```python
from build123d import *

# Parameters (mm, degrees)
CROQUIS1_W                       = 160
CROQUIS1_H                       = 140
CROQUIS1_R                       = 51.15
SALIENTE_EXTRUIR1_DEPTH          = 0.9
CROQUIS4_W                       = 20
CROQUIS4_H                       = 140
SALIENTE_EXTRUIR3_DEPTH          = 1
TALADRO_DE_MARGEN_PARA_M81_D     = 9
TALADRO_DE_MARGEN_PARA_M81_DEPTH = 10
TALADRO_DE_MARGEN_PARA_M81_TIP   = 2.703872786
SALIENTE_EXTRUIR4_DEPTH          = 21


with BuildPart() as part:
    # Croquis1 → Saliente-Extruir1 (new body)
    with BuildSketch(Plane(origin=(0, 0, 0), x_dir=(1, 0, 0), z_dir=(0, 1, 0))):
        Rectangle(CROQUIS1_W, CROQUIS1_H)
        with Locations(Location((0, 0, 0), (0, 0, 270))):
            Circle(CROQUIS1_R, mode=Mode.SUBTRACT)
    extrude(amount=SALIENTE_EXTRUIR1_DEPTH)

    # Croquis4 → Saliente-Extruir3 (add)
    with BuildSketch(Plane.XZ):
        with Locations((70, 0)):
            Rectangle(CROQUIS4_W, CROQUIS4_H)
        with Locations((-70, 0)):
            Rectangle(CROQUIS4_W, CROQUIS4_H)
    extrude(amount=SALIENTE_EXTRUIR3_DEPTH)

    # Taladro de margen para M81
    with Locations(Plane(origin=(-70, 0.9, -50), x_dir=(0, 0, 1), z_dir=(0, 1, 0))):
        with Locations((0, 0), (50, 0), (100, 0), (100, 140), (50, 140), (0, 140)):
            Hole(TALADRO_DE_MARGEN_PARA_M81_D / 2, depth=TALADRO_DE_MARGEN_PARA_M81_DEPTH)
            with Locations((0, 0, -(TALADRO_DE_MARGEN_PARA_M81_DEPTH + TALADRO_DE_MARGEN_PARA_M81_TIP / 2))):  # 118° drill point
                Cone(0, TALADRO_DE_MARGEN_PARA_M81_D / 2, TALADRO_DE_MARGEN_PARA_M81_TIP, mode=Mode.SUBTRACT)

    # Croquis5 → Saliente-Extruir4 (add)
    with BuildSketch(Plane.XZ):
        with BuildLine():
            ThreePointArc((57.15, 0), (0, 57.15), (-57.15, 0))
            Line((-57.15, 0), (-58.15, 0))
            ThreePointArc((-58.15, 0), (0, 58.15), (58.15, 0))
            Line((58.15, 0), (57.15, 0))
        make_face()
        with BuildLine():
            ThreePointArc((-58.141400912, -1), (0, -58.15), (58.141400912, -1))
            Line((58.141400912, -1), (57.141250424, -1))
            ThreePointArc((57.141250424, -1), (0, -57.15), (-57.141250424, -1))
            Line((-57.141250424, -1), (-58.141400912, -1))
        make_face()
    extrude(amount=-SALIENTE_EXTRUIR4_DEPTH)


solid = part.part
```
The model under review builds one solid part; all positions refer to its coordinate system, in mm. A direction names the side the tool comes from. Give positions to 0.01 mm unless a question says otherwise; leave off trailing zeros. Write each loop counter-clockwise with the first axis right and the second up, starting at its lowest first coordinate (ties: lowest second). Pieces come first, ordered by that corner, then holes. Notation, with made-up numbers: (20, -20.5) -> (37, -20.5) arc R18 ccw to (37, -6.5) -> close; hole circle Ø1 at (9.5, -36). An arc over 180 degrees is marked (long way). Put each result on its own line as item: value.
(1) Tool access review of faces 1 (the flat face through (41, 0, 32)), 2 (the cylindrical face through (1.257, 10.809, 57.136)), 3 (the cylindrical face through (-1.279, 10.809, 58.136)): name each direction out of +Z, -Z, +X, -X, +Y, -Y from which nothing blocks a thin tool from reaching the whole face with its end or side.
Results are:
face 1: +Z, -Z, -Y
face 2: +Y
face 3: +Z, +Y
(2) We need section B-B, the plane y = 4.75. Give the boundary of the cut face in (x, z).
Results are:
outline: (-58.15, 0) -> (-57.15, 0) arc R57.15 cw to (57.15, 0) -> (58.15, 0) arc R58.15 ccw to start; (-58.14, -1) arc R58.15 ccw to (58.14, -1) -> (57.14, -1) arc R57.15 cw to (-57.14, -1) -> close
(3) We need section C-C, the plane z = 2. Give the boundary of the cut face in (x, y) (3 decimals), and give its area (3 significant figures).
Results are:
outline: (-80, -1) -> (-74.031, -1) -> (-74.031, 0.9) -> (-80, 0.9) -> close; (-65.969, -1) -> (-60, -1) -> (-60, 0) -> (-51.111, 0) -> (-51.111, 0.9) -> (-57.115, 0.9) -> (-57.115, 21) -> (-58.116, 21) -> (-58.116, 0.9) -> (-65.969, 0.9) -> close; (51.111, 0) -> (60, 0) -> (60, -1) -> (65.969, -1) -> (65.969, 0.9) -> (58.116, 0.9) -> (58.116, 21) -> (57.115, 21) -> (57.115, 0.9) -> (51.111, 0.9) -> close; (74.031, -1) -> (80, -1) -> (80, 0.9) -> (74.031, 0.9) -> close
area: 102 mm²
(4) For pin 1 Ø4 at (y, z) = (13.5, 8.5) entering from -X; pin 2 Ø4 at (x, y) = (46.5, 11) entering from +Z; pin 3 Ø2 at (y, z) = (15.5, -51.5) entering from +X; pin 4 Ø7 at (x, z) = (70, 0) entering from +Y, all flat-tipped, find the tip position at first contact; note any pin that passes through.
Results are:
pin 1: x = -57.79
pin 2: z = 37.43
pin 3: x = 28.83
pin 4: through
(5) We need section A-A, the plane x = -70. Give the boundary of the cut face in (y, z).
Results are:
outline: (-1, -70) -> (0.9, -70) -> (0.9, -54.5) -> (-1, -54.5) -> close; (-1, -45.5) -> (0.9, -45.5) -> (0.9, -4.5) -> (-1, -4.5) -> close; (-1, 4.5) -> (0.9, 4.5) -> (0.9, 45.5) -> (-1, 45.5) -> close; (-1, 54.5) -> (0.9, 54.5) -> (0.9, 70) -> (-1, 70) -> close
(6) To check wall thickness, follow probe 1 along X at (y, z) = (-0.1, 0); probe 2 along Y at (x, z) = (49, -44.5); probe 3 along Z at (x, y) = (24, 17). State the ranges of each line that lie inside material, in increasing order. Write a range as from..to.
Results are:
probe 1: -80..-74.5, -65.5..-60, 60..65.5, 74.5..80
probe 2: 0..0.9
probe 3: -52.97..-51.87, 51.87..52.97
(7) We need section D-D, the plane x = 35. Give the boundary of the cut face in (y, z), and give its area (3 significant figures).
Results are:
outline: (0, -70) -> (0.9, -70) -> (0.9, -46.44) -> (21, -46.44) -> (21, -45.18) -> (0.9, -45.18) -> (0.9, -37.3) -> (0, -37.3) -> close; (0, 37.3) -> (0.9, 37.3) -> (0.9, 45.18) -> (21, 45.18) -> (21, 46.44) -> (0.9, 46.44) -> (0.9, 70) -> (0, 70) -> close
area: 109 mm²
